```python
from build123d import *

# Parameters (mm, degrees)
SKETCH1_R           = 1.5
BOSS_EXTRUDE1_DEPTH = 4


with BuildPart() as part:
    # Sketch1 → Boss-Extrude1 (new body)
    with BuildSketch(Plane.XY):
        with BuildLine():
            Line((18.283368275, 6.499999319), (6.716637678, 6.499999319))
            ThreePointArc((6.716637678, 6.499999319), (5.206858361, 6.239169805), (3.872099046, 5.486917725))
            Line((3.872099046, 5.486917725), (2.976e-06, 2.328161032))
            Line((2.976e-06, 2.328161032), (2.976e-06, -6.81e-07))
            Line((2.976e-06, -6.81e-07), (25.000002976, -6.81e-07))
            Line((25.000002976, -6.81e-07), (25.000002976, 2.328161032))
            Line((25.000002976, 2.328161032), (21.127906906, 5.486917725))
            ThreePointArc((21.127906906, 5.486917725), (19.793147591, 6.239169805), (18.283368275, 6.499999319))
        make_face()
        with Locations((7.050002976, 2.969999319)):
            Circle(SKETCH1_R, mode=Mode.SUBTRACT)
        with Locations((18.250002976, 2.969999319)):
            Circle(SKETCH1_R, mode=Mode.SUBTRACT)
    extrude(amount=BOSS_EXTRUDE1_DEPTH)


solid = part.part
```
Check sheet for the modelled part. Datum: model origin and axes. Units: mm. Coordinates: 2 decimals unless noted, no trailing zeros. Write each loop counter-clockwise with the first axis right and the second up, starting at its lowest first coordinate (ties: lowest second). Pieces come first, ordered by that corner, then holes. Notation, with made-up numbers: (-36.5, 61) -> (-21.5, 61) arc R22 cw to (-21.5, 90) -> close; hole circle Ø7 at (34.25, 12). An arc over 180 degrees is marked (long way). Use a Markdown table: item, result.
1. Release check for a two-part mould opening along X. For faces 1 (the cylindrical face through (5.227, 6.246, 1.972)), 2 (the flat face through (12, 3, 4)), 3 (the cylindrical face through (19.813, 6.232, 1.972)), 4 (the cylindrical face through (8.436, 2.395, 1.972)) record: pulls with the +X half, pulls with the -X half, needs draft (parallel to the pull), parting line crosses it, or undercut.
Reported:
| item | result |
|---|---|
| face 1 | pulls with the -X half |
| face 2 | needs draft |
| face 3 | pulls with the +X half |
| face 4 | undercut |
2. Sectioned sample at D-D (x = 18.5). Enter the section's corners in (y, z).
Reported:
| item | result |
|---|---|
| outline | (0, 0) -> (1.49, 0) -> (1.49, 4) -> (0, 4) -> close; (4.45, 0) -> (6.49, 0) -> (6.49, 4) -> (4.45, 4) -> close |
3. Sectioned sample at B-B (z = 3.4). Enter the section's corners in (x, y), plus the area to 3 significant figures.
Reported:
| item | result |
|---|---|
| outline | (0, 0) -> (25, 0) -> (25, 2.33) -> (21.13, 5.49) arc R4.5 ccw to (18.28, 6.5) -> (6.72, 6.5) arc R4.5 ccw to (3.87, 5.49) -> (0, 2.33) -> close; hole circle Ø3 at (7.05, 2.97); hole circle Ø3 at (18.25, 2.97) |
| area | 126 mm2 |
4. Go/stop test with flat-tipped pins: pin 1 Ø1.5 at (y, z) = (5.5, 1.5) entering from +X; pin 2 Ø1 at (y, z) = (5, 1) entering from +X; pin 3 Ø2.5 at (x, y) = (18.25, 2.97) entering from +Z. Record where each tip stops, or that it passes through.
Reported:
| item | result |
|---|---|
| pin 1 | stops at x = 22.03 |
| pin 2 | stops at x = 22.34 |
| pin 3 | passes through |
5. Sectioned sample at C-C (y = 2.97). Enter the section's corners in (x, z).
Reported:
| item | result |
|---|---|
| outline | (0.79, 0) -> (5.55, 0) -> (5.55, 4) -> (0.79, 4) -> close; (8.55, 0) -> (16.75, 0) -> (16.75, 4) -> (8.55, 4) -> close; (19.75, 0) -> (24.21, 0) -> (24.21, 4) -> (19.75, 4) -> close |
6. Scan lines: line 1 along X through (y, z) = (2.97, 1.7); line 2 along X through (y, z) = (3, 3.5); line 3 along Y through (x, z) = (19.25, 0.35). Record each from-to range of solid material in increasing order.
Reported:
| item | result |
|---|---|
| line 1 | x = 0.79 to 5.55, 8.55 to 16.75, 19.75 to 24.21 |
| line 2 | x = 0.82 to 5.55, 8.55 to 16.75, 19.75 to 24.18 |
| line 3 | y = 0 to 1.85, 4.09 to 6.39 |
7. Sectioned sample at A-A (x = 8.25). Enter the section's corners in (y, z).
Reported:
| item | result |
|---|---|
| outline | (0, 0) -> (2.07, 0) -> (2.07, 4) -> (0, 4) -> close; (3.87, 0) -> (6.5, 0) -> (6.5, 4) -> (3.87, 4) -> close |
